from build123d import *

# Parameters (mm, degrees)
SKETCH2_W               = 330.2
SKETCH2_H               = 330.2
BOSS_EXTRUDE1_DEPTH     = 177.8
CUT_EXTRUDE1_DEPTH      = 410.759551445
CUT_EXTRUDE1_DEPTH_BACK = 410.759551445
SKETCH3_R               = 21.59
SKETCH5_R               = 8.382
CUT_EXTRUDE3_DEPTH      = 101.6
SKETCH6_R               = 21.59
CUT_EXTRUDE4_DEPTH      = 165.1
FILLET1_R               = 5.08
FILLET2_R               = 25.4


with BuildPart() as part:
    # Sketch2 → Boss-Extrude1 (new body)
    with BuildSketch(Plane.XY):
        Rectangle(SKETCH2_W, SKETCH2_H)
    extrude(amount=BOSS_EXTRUDE1_DEPTH)

    # Sketch3 → Cut-Extrude1 (cut, two sides: drawn at the far end of the back side and taken through both)
    with BuildSketch(Plane(origin=(165.1, 0, 0), x_dir=(0, 0, -1), z_dir=(1, 0, 0)).offset(-CUT_EXTRUDE1_DEPTH_BACK)):
        with Locations((-101.6, 0)):
            Circle(SKETCH3_R)
    extrude(amount=CUT_EXTRUDE1_DEPTH + CUT_EXTRUDE1_DEPTH_BACK, mode=Mode.SUBTRACT)

    # Sketch5 → Cut-Extrude3 (cut)
    with BuildSketch(Plane(origin=(0, 0, 0), x_dir=(-1, 0, 0), z_dir=(0, 0, -1))):
        Circle(SKETCH5_R)
    extrude(amount=-CUT_EXTRUDE3_DEPTH, mode=Mode.SUBTRACT)

    # Sketch6 → Cut-Extrude4 (cut)
    with BuildSketch(Plane.XZ.offset(165.1)):
        with Locations(Location((0, 101.6, 0), (0, 0, 270))):
            Circle(SKETCH6_R)
    extrude(amount=-CUT_EXTRUDE4_DEPTH, mode=Mode.SUBTRACT)

    # Fillet1
    fillet1_edges = [part.edges().sort_by_distance(p)[0] for p in [
        (-165.1, 0, 177.8),
        (0, -165.1, 177.8),
        (165.1, 0, 177.8),
        (0, 165.1, 177.8),
    ]]
    fillet(fillet1_edges, radius=FILLET1_R)

    # Fillet2
    # the kernel refuses this fillet: 25.4 mm, written as the material it takes off along each edge
    with BuildSketch(Plane(origin=(-139.7, 139.7, 177.8), x_dir=(0, 1, 0), z_dir=(1, 0, 0))) as fillet2_piece_1:
        with BuildLine():
            CenterArc((20.32, -5.08), 5.08, 0, 90)
            Line((25.4, -5.08), (25.4, 0))
            Line((25.4, 0), (20.32, 0))
        make_face()
    revolve(axis=Axis((-139.7, 139.7, 177.8), (0, 0, 1)), revolution_arc=90, mode=Mode.SUBTRACT)
    with BuildSketch(Plane(origin=(139.7, 139.7, 177.8), x_dir=(1, 0, 0), z_dir=(0, -1, 0))) as fillet2_piece_2:
        with BuildLine():
            CenterArc((20.32, -5.08), 5.08, 0, 90)
            Line((25.4, -5.08), (25.4, 0))
            Line((25.4, 0), (20.32, 0))
        make_face()
    revolve(axis=Axis((139.7, 139.7, 177.8), (0, 0, 1)), revolution_arc=90, mode=Mode.SUBTRACT)
    with BuildSketch(Plane(origin=(-139.7, -139.7, 177.8), x_dir=(-1, 0, 0), z_dir=(0, 1, 0))) as fillet2_piece_3:
        with BuildLine():
            CenterArc((20.32, -5.08), 5.08, 0, 90)
            Line((25.4, -5.08), (25.4, 0))
            Line((25.4, 0), (20.32, 0))
        make_face()
    revolve(axis=Axis((-139.7, -139.7, 177.8), (0, 0, 1)), revolution_arc=90, mode=Mode.SUBTRACT)
    with BuildSketch(Plane(origin=(139.7, -139.7, 177.8), x_dir=(0, -1, 0), z_dir=(-1, 0, 0))) as fillet2_piece_4:
        with BuildLine():
            CenterArc((20.32, -5.08), 5.08, 0, 90)
            Line((25.4, -5.08), (25.4, 0))
            Line((25.4, 0), (20.32, 0))
        make_face()
    revolve(axis=Axis((139.7, -139.7, 177.8), (0, 0, 1)), revolution_arc=90, mode=Mode.SUBTRACT)
    with BuildSketch(Plane(origin=(165.1, -165.1, -63.5), x_dir=(-1, 0, 0), z_dir=(0, 0, 1)), Plane(origin=(165.1, 165.1, -63.5), x_dir=(0, -1, 0), z_dir=(0, 0, 1))) as fillet2_piece_5:
        with BuildLine():
            CenterArc((FILLET2_R, -FILLET2_R), FILLET2_R, 90, 90)
            Line((0, -FILLET2_R), (0, 0))
            Line((0, 0), (FILLET2_R, 0))
        make_face()
    extrude(amount=241.3, mode=Mode.SUBTRACT)
    with BuildSketch(Plane(origin=(-165.1, -165.1, -63.5), x_dir=(1, 0, 0), z_dir=(0, 0, 1)), Plane(origin=(-165.1, 165.1, -63.5), x_dir=(0, -1, 0), z_dir=(0, 0, 1))) as fillet2_piece_6:
        with BuildLine():
            CenterArc((FILLET2_R, FILLET2_R), FILLET2_R, 180, 90)
            Line((0, FILLET2_R), (0, 0))
            Line((0, 0), (FILLET2_R, 0))
        make_face()
    extrude(amount=241.3, mode=Mode.SUBTRACT)


solid = part.part
CAD build for the part. Positions are in the model's coordinates, mm. A direction names the side the tool comes from. Coordinates: 2 decimals unless noted, no trailing zeros. Write each loop counter-clockwise with the first axis right and the second up, starting at its lowest first coordinate (ties: lowest second). Pieces come first, ordered by that corner, then holes. Notation, with made-up numbers: M 4.5,54 L 27.5,54 A32 ccw 27.5,88 Z; hole C 67,-21.5 d11. An arc over 180 degrees is marked long. Answer as a JSON object with one key per item and string values. Group by question number.
1) Saw through at A-A (z = 101.6). Write the cut outline in (x, y).
2) Wall check: line 1 (Z direction, x = -35, y = 0); line 2 (X direction, y = -55, z = 101); line 3 (X direction, y = 0, z = 35). Give the ranges that are in metal, low to high. Write a range as from..to.
3) Mould opens along Y. For faces 1 (the face through (-2, 2, 177.8)), 2 (the face through (-2.311, 14.592, 117.513)), 3 (the face through (157.86, 157.46, 85.15)), 4 (the face through (157.46, -157.86, 85.15)) say: +Y half, -Y half, draft (parallel to the pull), parting line (faces both ways), or undercut.
4) Saw through at B-B (x = 26). Write the cut outline in (y, z), plus the area to 3 significant figures.
5) Tool access for faces 5 (the face through (-157.86, -157.46, 85.15)), 6 (the face through (-8.269, -83.706, 81.656)), 7 (the face through (-8, 2.5, 40.3)): list every direction of +Z, -Z, +X, -X, +Y, -Y with a clear straight run to the whole face (end or side of a thin tool).
Values follow:
{
 "1": {"outline": "M -165.1,-139.7 A25.4 ccw -139.7,-165.1 L -21.59,-165.1 L -21.59,-21.59 L -165.1,-21.59 Z; M -165.1,21.59 L 165.1,21.59 L 165.1,139.7 A25.4 ccw 139.7,165.1 L -139.7,165.1 A25.4 ccw -165.1,139.7 Z; M 21.59,-165.1 L 139.7,-165.1 A25.4 ccw 165.1,-139.7 L 165.1,-21.59 L 21.59,-21.59 Z"},
 "2": {"line 1": "z = 0..80.01, 123.19..177.8", "line 2": "x = -165.1..-21.58, 21.58..165.1", "line 3": "x = -165.1..-8.38, 8.38..165.1"},
 "3": {"face 1": "draft", "face 2": "undercut", "face 3": "+Y half", "face 4": "-Y half"},
 "4": {"outline": "M -165.1,0 L 165.1,0 L 165.1,172.72 A5.08 ccw 160.02,177.8 L -160.02,177.8 A5.08 ccw -165.1,172.72 Z; hole C 0,101.6 d43.18", "area": "57,200 mm2"},
 "5": {"face 5": "+Z, -Z, -X, -Y", "face 6": "-Y", "face 7": "-Z"}
}
